Could you check a few things on this drawing? It's one solid part, dimensions in mm from its lowest x, y, z. A direction names the side the tool comes from. Coordinates: 2 decimals unless noted, no trailing zeros. Write each loop counter-clockwise with the first axis right and the second up, starting at its lowest first coordinate (ties: lowest second). Pieces come first, ordered by that corner, then holes.
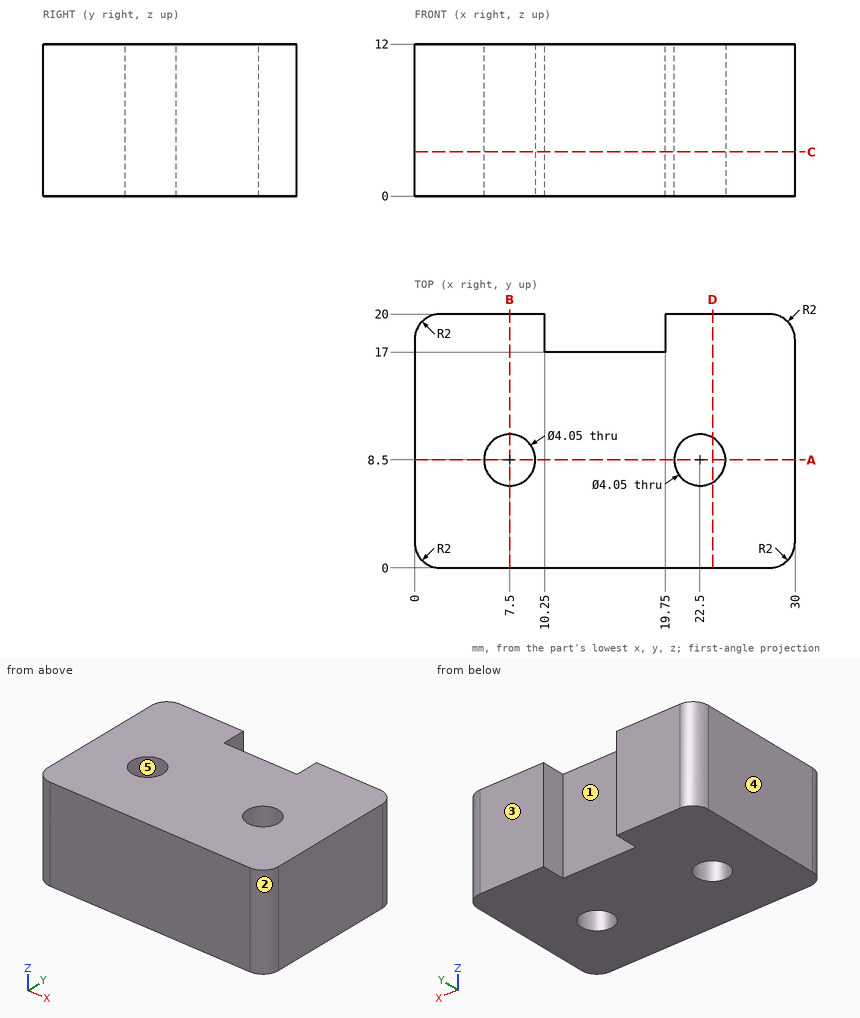
1) On a 3-axis mill with a long thin cutter (end or side, diameter ignored), from which of +Z, -Z, +X, -X, +Y, -Y can I reach the whole of each face in a straight line? I mean the marked faces 1 and 2. Say none if no direction works.
Values follow:
face 1: +Z, -Z, +Y
face 2: +Z, -Z, +X, -Y
2) Imagine slicing it at D-D on x = 23.5. Please give me the cut outline in (y, z).
Values follow:
outline: (0, 0) - (6.74, 0) - (6.74, 12) - (0, 12) - close; (10.26, 0) - (20, 0) - (20, 12) - (10.26, 12) - close
3) I need wall thicknesses on probe 1 along Y at (x, z) = (7.5, 6.25) (3 decimals); probe 2 along X at (y, z) = (17.75, 5.75); probe 3 along Y at (x, z) = (21.75, 10.25). Which ranges of each line are inside material? Lowest first, please.
Values follow:
probe 1: y = 0 to 6.475, 10.525 to 20
probe 2: x = 0 to 10.25, 19.75 to 30
probe 3: y = 0 to 6.62, 10.38 to 20
4) Will these pins go through, and if not, where does the flat tip stop? pin 1 (2 mm diameter, centred on x = 5, z = 1.5, fed in from -Y); pin 2 (5 mm diameter, centred on x = 13.5, z = 8, fed in from +Y).
Values follow:
pin 1: stops at y = 0
pin 2: stops at y = 17
5) We'd pull the mould along Y, two halves only. Please class the marked faces 3, 4 and 5: pulls with the +Y half, pulls with the -Y half, needs draft (parallel to the pull), parting line crosses it, or undercut.
Values follow:
face 3: pulls with the +Y half
face 4: needs draft
face 5: undercut
6) Imagine slicing it at C-C on z = 3.5. Please give me the cut outline in (x, y) (3 decimals).
Values follow:
outline: (0, 2) arc R2 ccw to (2, 0) - (28, 0) arc R2 ccw to (30, 2) - (30, 18) arc R2 ccw to (28, 20) - (19.75, 20) - (19.75, 17) - (10.25, 17) - (10.25, 20) - (2, 20) arc R2 ccw to (0, 18) - close; hole circle Ø4.05 at (7.5, 8.5); hole circle Ø4.05 at (22.5, 8.5)
7) Imagine slicing it at A-A on y = 8.5. Please give me the cut outline in (x, z) (3 decimals).
Values follow:
outline: (0, 0) - (5.475, 0) - (5.475, 12) - (0, 12) - close; (9.525, 0) - (20.475, 0) - (20.475, 12) - (9.525, 12) - close; (24.525, 0) - (30, 0) - (30, 12) - (24.525, 12) - close
8) Imagine slicing it at B-B on x = 7.5. Please give me the cut outline in (y, z) (3 decimals).
Values follow:
outline: (0, 0) - (6.475, 0) - (6.475, 12) - (0, 12) - close; (10.525, 0) - (20, 0) - (20, 12) - (10.525, 12) - close
